Verification items for the finished model (mm, model axes). A direction names the side the tool comes from. Round coordinates to 2 decimals unless told otherwise and drop trailing zeros. Write each loop counter-clockwise with the first axis right and the second up, starting at its lowest first coordinate (ties: lowest second). Pieces come first, ordered by that corner, then holes. Notation, with made-up numbers: M 7.25,7.5 L 62.25,7.5 A31 ccw 62.25,37.5 Z; hole C -13,79.25 d6. An arc over 180 degrees is marked long. One line per item, written item: value. Start each with the question number.
Item 1: Section check A-A, the plane y = 1.5. Record the cut outline in (x, z), then the cut area to 3 significant figures.
Item 2: Gauge pin test, flat ends, axial feed: pin 1 (0.5 mm diameter, centred on y = -1.5, z = 2, fed in from +X); pin 2 (1.9 mm diameter, centred on x = 0, z = 2.5, fed in from +Y); pin 3 (0.8 mm diameter, centred on y = 2.5, z = -0.5, fed in from -X). Record the tip position at first contact, or that the pin passes through.
Item 3: Tool access check on faces 1 (the face through (-2, 0, 2)), 2 (the face through (1.9, 1.9, -0.5)), 3 (the face through (-1.9, 1.9, -0.5)), 4 (the face through (-2, -2, 0)). Record the directions out of +Z, -Z, +X, -X, +Y, -Y that give a thin tool (end or side, any length) a straight path to the whole face; none if there is none.
Item 4: Section check B-B, the plane z = 2.25. Record the cut outline in (x, y), then the cut area to 3 significant figures.
Item 5: Thickness scan on probe 1 along Z at (x, y) = (3.75, -0.75); probe 2 along X at (y, z) = (0, 2.2); probe 3 along Z at (x, y) = (1.75, -1.5). Record the ranges inside material, lowest first. Write a range as from..to.
Item 6: Section check C-C, the plane y = -3. Record the cut outline in (x, z).
from build123d import *

# Parameters (mm, degrees)
SKETCH030_W  = 8
SKETCH030_H  = 8.8
PAD008_DEPTH = 1
PAD009_DEPTH = 2
FILLET015_R  = 1
SKETCH032_W  = 4
SKETCH032_H  = 8
PAD010_DEPTH = 2
FILLET016_R  = 0.25


with BuildPart() as part:
    # Sketch030 → Pad008 (new body)
    with BuildSketch(Plane.XY):
        Rectangle(SKETCH030_W, SKETCH030_H)
    extrude(amount=PAD008_DEPTH)

    # Sketch031 (on Face5 of Pad008) → Pad009 (join)
    with BuildSketch(Plane(origin=(0, 0, 0), x_dir=(1, 0, 0), z_dir=(0, 0, -1))):
        with BuildLine():
            ThreePointArc((1.9, 0.6), (0, 2.5), (-1.9, 0.6))
            Line((-1.9, 0.6), (-1.9, -4.4))
            Line((-1.9, -4.4), (1.9, -4.4))
            Line((1.9, 0.6), (1.9, -4.4))
        make_face()
    extrude(amount=PAD009_DEPTH)

    # Fillet015
    fillet015_edges = [part.edges().sort_by_distance(p)[0] for p in [
        (1.9, 1.9, -2),
        (0, -2.5, -2),
        (-1.9, 1.9, -2),
        (0, 4.4, -2),
    ]]
    fillet(fillet015_edges, radius=FILLET015_R)

    # Sketch032 (on Face6 of Pad008) → Pad010 (join)
    with BuildSketch(Plane.XY.offset(1)):
        Rectangle(SKETCH032_W, SKETCH032_H)
    extrude(amount=PAD010_DEPTH)

    # Fillet016
    fillet016_edges = [part.edges().sort_by_distance(p)[0] for p in [
        (-2, 4, 2),
        (2, 4, 2),
        (2, -4, 2),
        (-2, -4, 2),
        (-2, 0, 1),
        (0, 4, 1),
        (2, 0, 1),
        (0, -4, 1),
    ]]
    fillet(fillet016_edges, radius=FILLET016_R)


solid = part.part
Response values:
1. outline: M -4,0 L -1.9,0 L -1.9,-1 A1 ccw -0.9,-2 L 0.9,-2 A1 ccw 1.9,-1 L 1.9,0 L 4,0 L 4,1 L 2.25,1 A0.25 cw 2,1.25 L 2,3 L -2,3 L -2,1.25 A0.25 cw -2.25,1 L -4,1 Z
1. area: 23.2 mm2
2. pin 1: stops at x = 2
2. pin 2: stops at y = 4
2. pin 3: stops at x = -1.9
3. face 1: +Z, -X, +Y, -Y
3. face 2: -Z, +X, +Y, -Y
3. face 3: -Z, -X, +Y, -Y
3. face 4: -Z, -Y
4. outline: M -2,-3.75 A0.25 ccw -1.75,-4 L 1.75,-4 A0.25 ccw 2,-3.75 L 2,3.75 A0.25 ccw 1.75,4 L -1.75,4 A0.25 ccw -2,3.75 Z
4. area: 31.9 mm2
5. probe 1: z = 0..1
5. probe 2: x = -2..2
5. probe 3: z = 0..3
6. outline: M -4,0 L 4,0 L 4,1 L 2.25,1 A0.25 cw 2,1.25 L 2,3 L -2,3 L -2,1.25 A0.25 cw -2.25,1 L -4,1 Z
